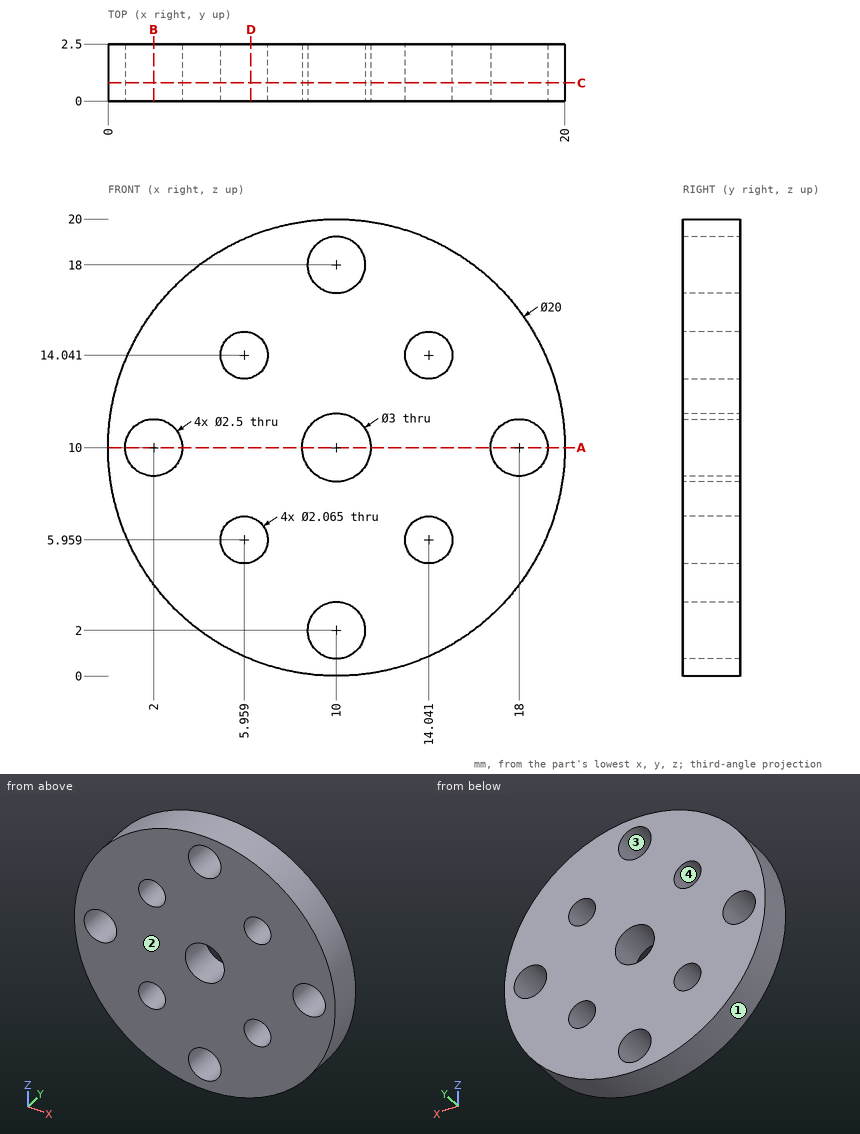
Drawing for the job (mm, zero at the part's lowest x, y, z). Round coordinates to 2 decimals unless told otherwise and drop trailing zeros. Write each loop counter-clockwise with the first axis right and the second up, starting at its lowest first coordinate (ties: lowest second). Pieces come first, ordered by that corner, then holes. Notation, with made-up numbers: (40, 44.25) - (58, 44.25) arc R16 cw to (58, 66.25) - close; hole circle Ø5 at (-3, 63). An arc over 180 degrees is marked (long way). Write item = value, one per line. Start each with the question number.
Q1. Band-saw the part on D-D (x = 6.25). Give the cut face in (y, z).
Q2. Band-saw the part on B-B (x = 2). Give the cut face in (y, z).
Q3. Band-saw the part on C-C (y = 0.8). Count the separate pieces of the cut face and the enclosed holes in it, then the cut area to 3 significant figures.
Q4. Drop flat-ended pins along their axis: pin 1 (1.7 mm diameter, centred on x = 14.04, z = 5.96, fed in from -Y); pin 2 (1.5 mm diameter, centred on x = 12, y = 0.5, fed in from -Z); pin 3 (1.5 mm diameter, centred on y = 1.5, z = 7.5, fed in from -X). Give the stop position or say it passes through.
Q5. Probe L1, parallel to X at y = 0.95, z = 10; L2, parallel to Z at x = 13.5, y = 1.95; L3, parallel to Z at x = 13.25, y = 2 (1 decimal). List the from-to ranges inside material, lowest first. Write a range as from..to.
Q6. Mould opens along X. For the marked faces 1, 2, 3 and 4 say: pulls with the +X half, pulls with the -X half, needs draft (parallel to the pull), parting line crosses it, or undercut.
Q7. Band-saw the part on A-A (z = 10). Give the cut face in (x, y), then the cut area to 3 significant figures.
Answers below:
q1.outline = (0, 0.73) - (2.5, 0.73) - (2.5, 4.97) - (0, 4.97) - close; (0, 6.95) - (2.5, 6.95) - (2.5, 13.05) - (0, 13.05) - close; (0, 15.03) - (2.5, 15.03) - (2.5, 19.27) - (0, 19.27) - close
q2.outline = (0, 4) - (2.5, 4) - (2.5, 8.75) - (0, 8.75) - close; (0, 11.25) - (2.5, 11.25) - (2.5, 16) - (0, 16) - close
q3.separate_pieces = 1
q3.enclosed_holes = 9
q3.area = 274 mm2
q4.pin_1 = through
q4.pin_2 = 0.08
q4.pin_3 = 0.15
q5.L1 = 0..0.75, 3.25..8.5, 11.5..16.75, 19.25..20
q5.L2 = 0.63..5.08, 6.84..13.16, 14.92..19.37
q5.L3 = 0.5..5.3, 6.6..13.4, 14.7..19.5
q6.face_1 = parting line crosses it
q6.face_2 = needs draft
q6.face_3 = undercut
q6.face_4 = undercut
q7.outline = (0, 0) - (0.75, 0) - (0.75, 2.5) - (0, 2.5) - close; (3.25, 0) - (8.5, 0) - (8.5, 2.5) - (3.25, 2.5) - close; (11.5, 0) - (16.75, 0) - (16.75, 2.5) - (11.5, 2.5) - close; (19.25, 0) - (20, 0) - (20, 2.5) - (19.25, 2.5) - close
q7.area = 30.0 mm2
